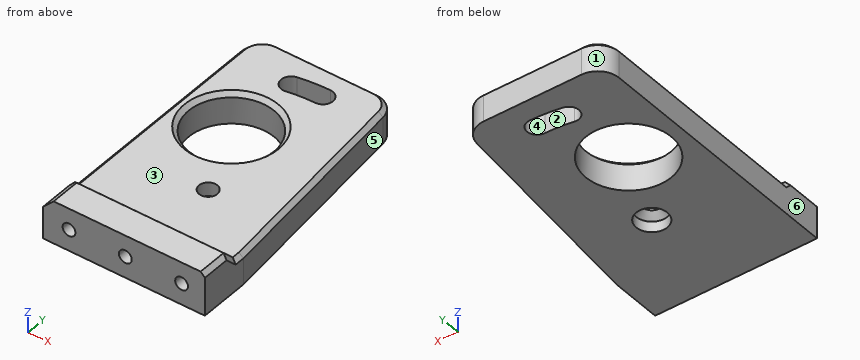
from build123d import *

# Parameters (mm, degrees)
AUFSATZ_LINEAR_AUSTRAGEN1_DEPTH      = 10
SKIZZE2_R                            = 1.5
SCHNITT_LINEAR_AUSTRAGEN1_DEPTH      = 8
SCHNITT_LINEAR_AUSTRAGEN3_DEPTH      = 2.8
SCHNITT_LINEAR_AUSTRAGEN5_DEPTH      = 72.591285383
SCHNITT_LINEAR_AUSTRAGEN5_DEPTH_BACK = 72.591285383
SKIZZE7_R                            = 10
FASE1_SIZE                           = 3
SCHNITT_LINEAR_AUSTRAGEN4_DEPTH      = 10
VERRUNDUNG1_R                        = 5
FASE2_SIZE                           = 1
FASE3_SIZE                           = 2.5
SKIZZE9_R                            = 2.15
SCHNITT_LINEAR_AUSTRAGEN7_DEPTH      = 71.291034025
SKIZZE10_R                           = 3.65
SCHNITT_LINEAR_AUSTRAGEN8_DEPTH      = 2.5
FASE4_SIZE                           = 1.5
SCHNITT_LINEAR_AUSTRAGEN9_DEPTH      = 10


# Some blends are built 0.0001 mm under size
with BuildPart() as part:
    # Skizze1 → Aufsatz-Linear austragen1 (new body)
    with BuildSketch(Plane.XY):
        Polygon((28.287001282, 57.370618027), (28.287001282, 0), (-13.088781156, 0), (-13.088781156, 27.348243657), (-13.088781156, 53.715647777), (-13.088781156, 57.370618027), (-13.088781156, 65.370618027), (28.287001282, 65.370618027), align=None)
    extrude(amount=AUFSATZ_LINEAR_AUSTRAGEN1_DEPTH)

    # Skizze2 → Schnitt-Linear austragen1 (cut)
    with BuildSketch(Plane.XZ):
        with Locations((-7, 5)):
            Circle(SKIZZE2_R)
        with Locations((6.18, 5)):
            Circle(SKIZZE2_R)
        with Locations((19.36, 5)):
            Circle(SKIZZE2_R)
    extrude(amount=-SCHNITT_LINEAR_AUSTRAGEN1_DEPTH, mode=Mode.SUBTRACT)

    # Skizze4 → Schnitt-Linear austragen3 (cut)
    with BuildSketch(Plane.XY.offset(10)):
        Polygon((-15.095168359, 10), (28.287001282, 10), (36.093332102, 46.989971623), (30.429094825, 65.957451721), (-16.081030445, 65.957451721), (-16.081030445, 27.753515123), align=None)
    extrude(amount=-SCHNITT_LINEAR_AUSTRAGEN3_DEPTH, mode=Mode.SUBTRACT)

    # Skizze7 → Schnitt-Linear austragen5 (cut, two sides: drawn at the far end of the back side and taken through both)
    with BuildSketch(Plane.XY.offset(7.2).offset(-SCHNITT_LINEAR_AUSTRAGEN5_DEPTH_BACK)):
        with Locations((-0.088781156, 40.531945717)):
            Circle(SKIZZE7_R)
    extrude(amount=SCHNITT_LINEAR_AUSTRAGEN5_DEPTH + SCHNITT_LINEAR_AUSTRAGEN5_DEPTH_BACK, mode=Mode.SUBTRACT)

    # Fase1
    # the kernel refuses this chamfer: 3 mm, written as the material it takes off along each edge
    with BuildSketch(Plane(origin=(-20.80383012, 10, 10), x_dir=(0, -0.9996219169112969, 0.027495876610586202), z_dir=(1, 0, 0))) as fase1_piece_1_section:
        Polygon((FASE1_SIZE * 0.999621916911, FASE1_SIZE * 0.0274958766106), (-FASE1_SIZE * 0.0274958766106, FASE1_SIZE * 0.999621916911), (0, 0), align=None)
    fase1_piece_1 = extrude(amount=56.805880365, mode=Mode.PRIVATE)
    fase1_piece_1 = split(fase1_piece_1, bisect_by=Plane(origin=(7.599110063, 8.999392985, 7.2), z_dir=(0, 0, 1)), keep=Keep.TOP, mode=Mode.PRIVATE)
    add(fase1_piece_1, mode=Mode.SUBTRACT)

    # Skizze5 → Schnitt-Linear austragen4 (cut)
    with BuildSketch(Plane(origin=(0, 0, 0), x_dir=(-1, 0, 0), z_dir=(0, 0, -1))):
        Polygon((-24.81273389, 11.736777957), (-19.336036603, 65.370618027), (-28.287001282, 65.370618027), (-28.287001282, 0), (-24.81273389, 0), align=None)
    extrude(amount=-SCHNITT_LINEAR_AUSTRAGEN4_DEPTH, mode=Mode.SUBTRACT)

    # Verrundung1
    verrundung1_edges = [part.edges().sort_by_distance(p)[0] for p in [
        (-13.088781156, 65.370618027, 3.6),
        (19.336036603, 65.370618027, 3.6),
    ]]
    fillet(verrundung1_edges, radius=VERRUNDUNG1_R)

    # Fase2
    fase2_edges = [part.edges().sort_by_distance(p)[0] for p in [
        (-13.088781156, 35.085309014, 7.2),
        (3.365909563, 65.370618027, 7.2),
        (22.303734377, 36.307659198, 7.2),
        (18.17174844, 64.081386954, 7.2),
        (-11.624315062, 63.906151933, 7.2),
        (-10.088781156, 40.531945717, 7.2),
        (-13.088781156, 8.4, 8.6),
        (24.81273389, 8.4, 8.6),
        (24.81273389, 10.768388979, 7.2),
        (24.81273389, 3.5, 10),
    ]]
    chamfer(fase2_edges, length=FASE2_SIZE)

    # Fase3
    fase3_edges = [part.edges().sort_by_distance(p)[0] for p in [
        (-13.088781156, 2.792893219, 10),
    ]]
    chamfer(fase3_edges, length=FASE3_SIZE)

    # Skizze9 → Schnitt-Linear austragen7 (cut, through all)
    with BuildSketch(Plane.XY.offset(7.2)):
        with Locations((7.911218844, 58.031945717)):
            Circle(SKIZZE9_R)
        with Locations((7.911218844, 23.031945717)):
            Circle(SKIZZE9_R)
    extrude(amount=-SCHNITT_LINEAR_AUSTRAGEN7_DEPTH, mode=Mode.SUBTRACT)

    # Skizze10 → Schnitt-Linear austragen8 (cut)
    with BuildSketch(Plane(origin=(0, 0, 0), x_dir=(-1, 0, 0), z_dir=(0, 0, -1))):
        with Locations((-7.911218844, 23.031945717)):
            Circle(SKIZZE10_R)
    extrude(amount=-SCHNITT_LINEAR_AUSTRAGEN8_DEPTH, mode=Mode.SUBTRACT)

    # Fase4
    fase4_edges = [part.edges().sort_by_distance(p)[0] for p in [
        (5.761218844, 23.031945717, 2.5),
    ]]
    chamfer(fase4_edges, length=FASE4_SIZE - 0.0001)  # a hair under: the kernel refuses the full size

    # Skizze11 → Schnitt-Linear austragen9 (cut)
    with BuildSketch(Plane.XY.offset(7.2)):
        with BuildLine():
            ThreePointArc((7.911218844, 60.381945717), (4.210709496, 60.198176768), (0.546614537, 59.648678277))
            ThreePointArc((0.546614537, 59.648678277), (-1.293880815, 56.88144557), (1.473351893, 55.040950218))
            ThreePointArc((1.473351893, 55.040950218), (4.676369307, 55.521301643), (7.911218844, 55.681945717))
            ThreePointArc((7.911218844, 55.681945717), (10.261218844, 58.031945717), (7.911218844, 60.381945717))
        make_face()
    extrude(amount=-SCHNITT_LINEAR_AUSTRAGEN9_DEPTH, mode=Mode.SUBTRACT)


solid = part.part
For this review, take the finished solid that the model builds, in its own axes (mm). Face numbers are marked on the shaded views. A direction names the side the tool comes from. Give positions to 0.01 mm unless a question says otherwise; leave off trailing zeros. Order: outer loops, then holes, each group sorted by start corner. A loop starts at its lowest first (then second) coordinate and runs counter-clockwise, first axis right, second up. Notation, with made-up numbers: M -24.5,-2 L -14.5,-2 A18 ccw -14.5,20 Z; hole C -21.75,13 d5. An arc over 180 degrees is marked long. Answer in a Markdown table with one row per item. Add a question column.
(1) Wall thickness on probe 1 along Z at (x, y) = (6.18, 2); probe 2 along X at (y, z) = (3, 5.75); probe 3 along Y at (x, z) = (6, 7): over which ranges is each line inside the solid? List them lowest first. Write a range as [from, to].
(2) For the marked faces 1 and 2, list the 3-axis set-ups (+Z, -Z, +X, -X, +Y, -Y) from which the entire face can be reached by the end or side of a thin tool; tool diameter is ignored.
(3) Consider section C-C on x = 6.5. Give the number of separate pieces and of enclosed holes in the cut face, and give its area (3 significant figures).
(4) Consider section B-B on y = 14.5. State the section outline as (x, z) points, and give its area (3 significant figures).
(5) Consider section A-A on z = 5. State the section outline as (x, y) points, and give its area (3 significant figures).
(6) For pin 1 (9.5 mm diameter, centred on x = 7.91, y = 23.03, fed in from +Z); pin 2 (2 mm diameter, centred on x = 8.5, y = 21.5, fed in from -Z); pin 3 (1 mm diameter, centred on x = -3, z = 9, fed in from +Y), all flat-tipped, find the tip position at first contact; note any pin that passes through.
(7) Mouldability with a two-part tool opening along X and no side actions: class the marked faces 3, 4, 5 and 6 as +X half, -X half, draft (parallel to the pull), parting line (faces both ways), or undercut.
Evaluation:
| question | item | result |
|---|---|---|
| 1 | probe 1 | z = [0, 3.5], [6.5, 10] |
| 1 | probe 2 | x = [-13.09, -8.3], [-5.7, 4.88], [7.48, 18.06], [20.66, 24.81] |
| 1 | probe 3 | y = [0, 22.05], [24.02, 31.61], [49.45, 55.63], [60.33, 64.57] |
| 2 | face 1 | +Z, -Z, -X, +Y |
| 2 | face 2 | +Z, -Z |
| 3 | separate pieces | 4 |
| 3 | enclosed holes | 0 |
| 3 | area | 292 mm^2 |
| 4 | outline | M -13.09,0 L 24.53,0 L 24.53,6.2 L 23.53,7.2 L -12.09,7.2 L -13.09,6.2 Z |
| 4 | area | 270 mm^2 |
| 5 | outline | M -13.09,0 L -8.5,0 L -8.5,8 L -5.5,8 L -5.5,0 L 4.68,0 L 4.68,8 L 7.68,8 L 7.68,0 L 17.86,0 L 17.86,8 L 20.86,8 L 20.86,0 L 24.81,0 L 24.81,11.74 L 19.79,60.88 A5 ccw 14.82,65.37 L -8.09,65.37 A5 ccw -13.09,60.37 Z; hole C -0.09,40.53 d20; hole M 0.55,59.65 A2.35 ccw 1.47,55.04 A32.65 cw 7.91,55.68 A2.35 ccw 7.91,60.38 A37.35 ccw Z; hole C 7.91,23.03 d4.3 |
| 5 | area | 1,870 mm^2 |
| 6 | pin 1 | stops at z = 7.2 |
| 6 | pin 2 | stops at z = 3.51 |
| 6 | pin 3 | stops at y = 8.5 |
| 7 | face 3 | draft |
| 7 | face 4 | undercut |
| 7 | face 5 | +X half |
| 7 | face 6 | -X half |
